The listing builds one solid part. Answer for the finished solid, in the listing's coordinates (mm). Round coordinates to 2 decimals unless told otherwise and drop trailing zeros. Loops run counter-clockwise (first coordinate to the right, second up) from the corner with the lowest first, then second, coordinate; pieces in that order, holes last. Notation, with made-up numbers: (66.5, -24) -> (120.5, -24) arc R16 ccw to (120.5, -14) -> close; hole circle Ø4 at (48.5, -16). An arc over 180 degrees is marked (long way). Use a Markdown table: item, result. Add a question column.
Q1. Section A-A on x = 3 is taken. Give the vertices of the cut face in (y, z).
Q2. Section D-D on z = 0.6 is taken. Give the vertices of the cut face in (x, y), then the cut area to 3 significant figures.
Q3. Consider line 1 (X direction, y = 3, z = 0.55); line 2 (Y direction, x = 26, z = 1.55). Determine where each line is inside the solid, lowest interval first.
Q4. Given pin 1 Ø5 at (x, y) = (3, 3) entering from +Z, flat-ended and moving along its own axis, determine where the tip first touches the part or whether it passes through.
Q5. For a pull along Y with two mould halves and no side action, classify faces 1 (the flat face through (27, 0, 1)), 2 (the flat face through (21, 28, 0)), 3 (the cylindrical face through (50.38, 3.21, 0.49)) as released by +Y, released by -Y, zero draft, split by the parting line, or undercut.
Q6. Section C-C on x = 27.5 is taken. Give the vertices of the cut face in (y, z), then the cut area to 3 significant figures.
from build123d import *

# Parameters (mm, degrees)
SKETCH1_W                                 = 55
SKETCH1_H                                 = 55
BOSS_EXTRUDE1_DEPTH                       = 2
SKETCH3_R                                 = 3.1
CUT_EXTRUDE1_DEPTH                        = 78.807454656
CSK_FOR_4_FLAT_HEAD_MACHINE_SCREW_2_COUNT = 2
CSK_FOR_4_FLAT_HEAD_MACHINE_SCREW_2_PITCH = 49
CSK_FOR_4_FLAT_HEAD_MACHINE_SCREW_3_COUNT = 2
CSK_FOR_4_FLAT_HEAD_MACHINE_SCREW_3_PITCH = 69.296464556
CSK_FOR_4_FLAT_HEAD_MACHINE_SCREW_4_COUNT = 2
CSK_FOR_4_FLAT_HEAD_MACHINE_SCREW_4_PITCH = 49


with BuildPart() as part:
    # Sketch1 → Boss-Extrude1 (new body)
    with BuildSketch(Plane.XY):
        with Locations((27.5, 27.5)):
            Rectangle(SKETCH1_W, SKETCH1_H)
    extrude(amount=BOSS_EXTRUDE1_DEPTH)

    # Sketch3 → Cut-Extrude1 (cut, through all)
    with BuildSketch(Plane.XY.offset(2)):
        with Locations((27.5, 27.5)):
            Circle(SKETCH3_R)
    extrude(amount=-CUT_EXTRUDE1_DEPTH, mode=Mode.SUBTRACT)

    # Sketch5 → CSK for #4 Flat Head Machine Screw (100)1 (revolve, cut)
    with BuildSketch(Plane(origin=(3, 52, 2), x_dir=(0, -1, 0), z_dir=(1, 0, 0))):
        Polygon((0, 0), (0, 2), (1.63195, 2), (1.63195, 1.028358553), (2.8575, 0), align=None)
    csk_for_4_flat_head_machine_screw_100 = revolve(axis=Axis((3, 52, 8.35), (0, 0, -1)), mode=Mode.SUBTRACT)

    # CSK for _4 Flat Head Machine Screw _ 2: CSK for #4 Flat Head Machine Screw (100)1 ×2
    with Locations(*[(i * CSK_FOR_4_FLAT_HEAD_MACHINE_SCREW_2_PITCH, 0, 0) for i in range(1, CSK_FOR_4_FLAT_HEAD_MACHINE_SCREW_2_COUNT)]):
        add(csk_for_4_flat_head_machine_screw_100, mode=Mode.SUBTRACT)

    # CSK for _4 Flat Head Machine Screw _ 3: CSK for #4 Flat Head Machine Screw (100)1 ×2
    with Locations(*[Vector(0.7071067811865477, -0.7071067811865475, 0) * (i * CSK_FOR_4_FLAT_HEAD_MACHINE_SCREW_3_PITCH) for i in range(1, CSK_FOR_4_FLAT_HEAD_MACHINE_SCREW_3_COUNT)]):
        add(csk_for_4_flat_head_machine_screw_100, mode=Mode.SUBTRACT)

    # CSK for _4 Flat Head Machine Screw _ 4: CSK for #4 Flat Head Machine Screw (100)1 ×2
    with Locations(*[(0, -i * CSK_FOR_4_FLAT_HEAD_MACHINE_SCREW_4_PITCH, 0) for i in range(1, CSK_FOR_4_FLAT_HEAD_MACHINE_SCREW_4_COUNT)]):
        add(csk_for_4_flat_head_machine_screw_100, mode=Mode.SUBTRACT)


solid = part.part
Checked values:
| question | item | result |
|---|---|---|
| 1 | outline | (0, 0) -> (1.37, 0) -> (1.37, 0.97) -> (0.14, 2) -> (0, 2) -> close; (4.63, 0) -> (50.37, 0) -> (50.37, 0.97) -> (49.14, 2) -> (5.86, 2) -> (4.63, 0.97) -> close; (53.63, 0) -> (55, 0) -> (55, 2) -> (54.86, 2) -> (53.63, 0.97) -> close |
| 2 | outline | (0, 0) -> (55, 0) -> (55, 55) -> (0, 55) -> close; hole circle Ø3.26 at (3, 3); hole circle Ø3.26 at (3, 52); hole circle Ø6.2 at (27.5, 27.5); hole circle Ø3.26 at (52, 3); hole circle Ø3.26 at (52, 52) |
| 2 | area | 2,960 mm2 |
| 3 | line 1 | x = 0 to 1.37, 4.63 to 50.37, 53.63 to 55 |
| 3 | line 2 | y = 0 to 24.79, 30.21 to 55 |
| 4 | pin 1 | stops at z = 1.7 |
| 5 | face 1 | released by -Y |
| 5 | face 2 | zero draft |
| 5 | face 3 | undercut |
| 6 | outline | (0, 0) -> (24.4, 0) -> (24.4, 2) -> (0, 2) -> close; (30.6, 0) -> (55, 0) -> (55, 2) -> (30.6, 2) -> close |
| 6 | area | 97.6 mm2 |
